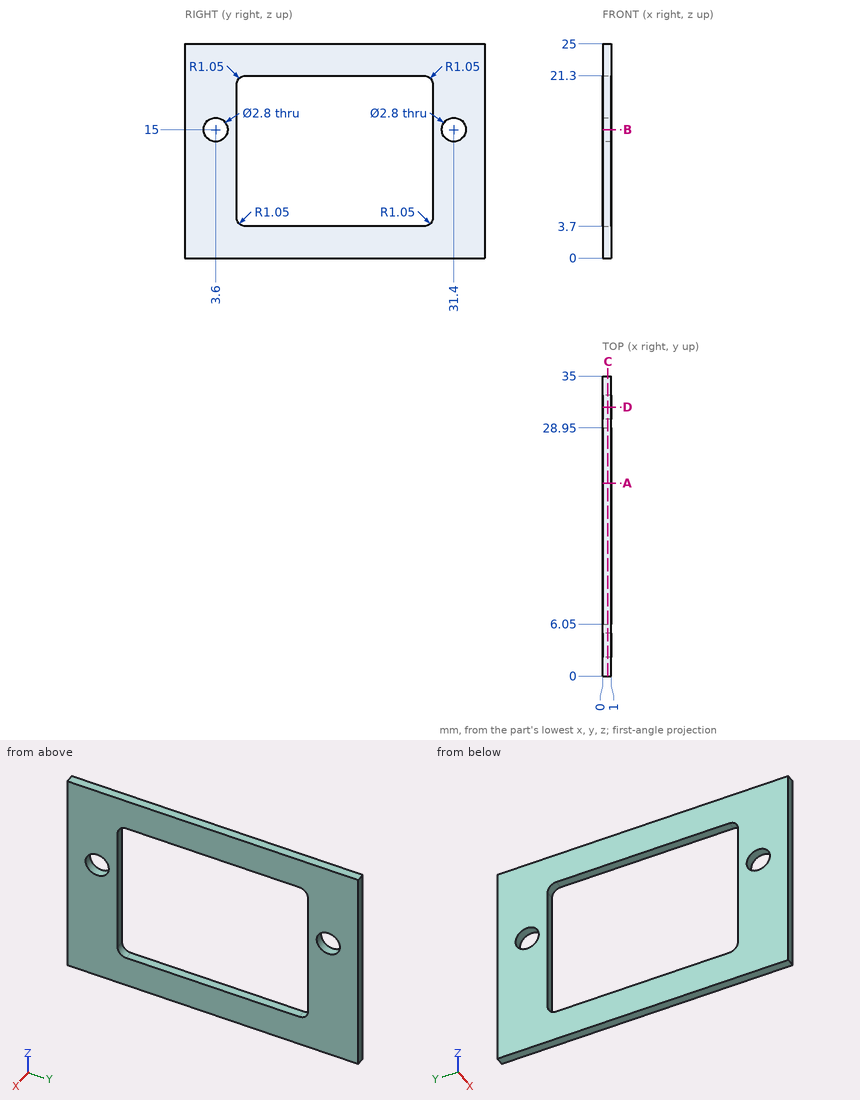
Check sheet for the drawn part. Datum: minimum x, y, z corner. Units: mm. Give positions to 0.01 mm unless a question says otherwise; leave off trailing zeros. Write each loop counter-clockwise with the first axis right and the second up, starting at its lowest first coordinate (ties: lowest second). Pieces come first, ordered by that corner, then holes. Notation, with made-up numbers: M -36.75,79 L -10.75,79 A14 ccw -10.75,102 Z; hole C 58.5,24.25 d8. An arc over 180 degrees is marked long. One line per question, with ' | ' between items.
1. Scan lines: line 1 along Y through (x, z) = (0.35, 15); line 2 along Z through (x, y) = (0.1, 8); line 3 along Y through (x, z) = (0.6, 11). Record each from-to range of solid material in increasing order. Write a range as from..to.
Ans:
line 1: 0..2.2, 5..6.05, 28.95..30, 32.8..35 | line 2: 0..3.7, 21.3..25 | line 3: 0..6.05, 28.95..35
2. Cross-section at D-D (y = 31.4). Enter the section's corners in (x, z), plus the area to 3 significant figures.
Ans:
outline: M 0,0 L 1,0 L 1,13.6 L 0,13.6 Z; M 0,16.4 L 1,16.4 L 1,25 L 0,25 Z | area: 22.2 mm2
3. Cross-section at C-C (x = 0.6). Enter the section's corners in (y, z).
Ans:
outline: M 0,0 L 35,0 L 35,25 L 0,25 Z; hole C 3.6,15 d2.8; hole M 6.05,4.75 A1.05 ccw 7.1,3.7 L 27.9,3.7 A1.05 ccw 28.95,4.75 L 28.95,20.25 A1.05 ccw 27.9,21.3 L 7.1,21.3 A1.05 ccw 6.05,20.25 Z; hole C 31.4,15 d2.8
4. Cross-section at B-B (z = 15). Enter the section's corners in (x, y), plus the area to 3 significant figures.
Ans:
outline: M 0,0 L 1,0 L 1,2.2 L 0,2.2 Z; M 0,5 L 1,5 L 1,6.05 L 0,6.05 Z; M 0,28.95 L 1,28.95 L 1,30 L 0,30 Z; M 0,32.8 L 1,32.8 L 1,35 L 0,35 Z | area: 6.50 mm2
5. Cross-section at A-A (y = 22.5). Enter the section's corners in (x, z), plus the area to 3 significant figures.
Ans:
outline: M 0,0 L 1,0 L 1,3.7 L 0,3.7 Z; M 0,21.3 L 1,21.3 L 1,25 L 0,25 Z | area: 7.40 mm2
